```python
from build123d import *

# Parameters (mm, degrees)
ESBO_O1_W                = 19
ESBO_O1_H                = 19
RESSALTO_EXTRUS_O1_DEPTH = 260
CASCA2_T                 = -1
ESBO_O2_R                = 3
CORTE_EXTRUS_O1_DEPTH    = 20


with BuildPart() as part:
    # Esboço1 → Ressalto-extrusão1 (new body)
    with BuildSketch(Plane.XY):
        Rectangle(ESBO_O1_W, ESBO_O1_H)
    extrude(amount=RESSALTO_EXTRUS_O1_DEPTH)

    # Casca2
    casca2_openings = [part.faces().sort_by_distance(p)[0] for p in [
        (0, 0, 260),
        (0, 0, 0),
    ]]
    offset(amount=CASCA2_T, openings=casca2_openings, kind=Kind.INTERSECTION)

    # Esboço2 → Corte-extrusão1 (cut, through all)
    with BuildSketch(Plane(origin=(0, 9.5, 0), x_dir=(1, 0, 0), z_dir=(0, 1, 0))):
        with Locations((0, -220.5)):
            Circle(ESBO_O2_R)
        with Locations((0, -245.5)):
            Circle(ESBO_O2_R)
        with Locations((0, -14.5)):
            Circle(ESBO_O2_R)
        with Locations((0, -39.5)):
            Circle(ESBO_O2_R)
    extrude(amount=-CORTE_EXTRUS_O1_DEPTH, mode=Mode.SUBTRACT)


solid = part.part
```
The model under review builds one solid part; all positions refer to its coordinate system, in mm. A direction names the side the tool comes from. Give positions to 0.01 mm unless a question says otherwise; leave off trailing zeros. Write each loop counter-clockwise with the first axis right and the second up, starting at its lowest first coordinate (ties: lowest second). Pieces come first, ordered by that corner, then holes. Notation, with made-up numbers: M 78,-32 L 88,-32 A9 ccw 88,-21 Z; hole C 23.25,4 d9. An arc over 180 degrees is marked long. Write item = value, one per line. Start each with the question number.
Q1. For line 1 (Z direction, x = 0, y = -8.9); line 2 (X direction, y = -1.5, z = 55), list the stretches that pass through material, from the lowest coordinate up.
Q2. Machinability: for faces 5 (the face through (-0.391, -8.993, 217.526)), 6 (the face through (0, -8.5, 128)), which of the approach directions +Z, -Z, +X, -X, +Y, -Y give a long, thin tool a straight path to every point of the face, cutting with its end or side? Answer none if there is none.
Q3. Clearance check with a flat-ended pin moving along its axis: pin 1 (5 mm diameter, centred on x = 0, z = 14.5, fed in from -Y). State where the tip first meets the part, or that it passes through.
Q4. Mouldability with a two-part tool opening along Z and no side actions: class faces 1 (the face through (-1, -9, 260)), 2 (the face through (-0.65, 9.01, 17.43)), 3 (the face through (0, 8.5, 128)), 4 (the face through (-0.391, -8.993, 242.526)) as released by +Z, released by -Z, zero draft, split by the parting line, or undercut.
Q5. We need section C-C (z = 220.5). State the section outline as (x, y) points.
Q6. We need section B-B (z = 51). State the section outline as (x, y) points, plus the area to 3 significant figures.
Q7. We need section A-A (y = -2). State the section outline as (x, z) points.
Result set:
q1.line_1 = 0 to 11.5, 17.5 to 36.5, 42.5 to 217.5, 223.5 to 242.5, 248.5 to 260
q1.line_2 = -9.5 to -8.5, 8.5 to 9.5
q2.face_5 = +Y, -Y
q2.face_6 = +Z, -Z
q3.pin_1 = through
q4.face_1 = released by +Z
q4.face_2 = undercut
q4.face_3 = zero draft
q4.face_4 = undercut
q5.outline = M -9.5,-9.5 L -3,-9.5 L -3,-8.5 L -8.5,-8.5 L -8.5,8.5 L -3,8.5 L -3,9.5 L -9.5,9.5 Z; M 3,-9.5 L 9.5,-9.5 L 9.5,9.5 L 3,9.5 L 3,8.5 L 8.5,8.5 L 8.5,-8.5 L 3,-8.5 Z
q6.outline = M -9.5,-9.5 L 9.5,-9.5 L 9.5,9.5 L -9.5,9.5 Z; hole M -8.5,-8.5 L 8.5,-8.5 L 8.5,8.5 L -8.5,8.5 Z
q6.area = 72.0 mm2
q7.outline = M -9.5,0 L -8.5,0 L -8.5,260 L -9.5,260 Z; M 8.5,0 L 9.5,0 L 9.5,260 L 8.5,260 Z
